Can you work these out from the model? Positions are in its coordinate system, mm. A direction names the side the tool comes from. Coordinates: 2 decimals unless noted, no trailing zeros. Write each loop counter-clockwise with the first axis right and the second up, starting at its lowest first coordinate (ties: lowest second). Pieces come first, ordered by that corner, then holes.
```python
from build123d import *

# Parameters (mm, degrees)
CUT_EXTRUDE_START   = -20
SKETCH_2_R          = 35
CUT_EXTRUDE_1_DEPTH = 20


with BuildPart() as part:
    # Эскиз1 → Повернуть1 (revolve)
    with BuildSketch(Plane.XY, mode=Mode.PRIVATE) as revolve_1_sk:
        Polygon((0, 0), (-35, 0), (-35, 15), (-120, 15), (-120, 10), (-40, 10), (-40, -30), (0, -30), align=None)
    revolve(revolve_1_sk.sketch.rotate(Axis((0, -30, 0), (0, 1, 0)), 270), axis=Axis((0, -30, 0), (0, 1, 0)))

    # Эскиз2 → Вырез-Вытянуть1 (cut)
    with BuildSketch(Plane.XZ.offset(30).offset(CUT_EXTRUDE_START)):
        with Locations(Location((0, 0, 0), (0, 0, 270))):
            Circle(SKETCH_2_R)
    extrude(amount=CUT_EXTRUDE_1_DEPTH, mode=Mode.SUBTRACT)


solid = part.part
```
1. If we section it at A-A, the plane y = -18: List the corners of the cut face in (x, z) for me, plus the area to 3 significant figures.
2. If we section it at D-D, the plane x = 65: List the corners of the cut face in (y, z) for me.
3. If we section it at C-C, the plane z = -4: List the corners of the cut face in (x, y) for me, plus the area to 3 significant figures.
4. Which directions (+Z, -Z, +X, -X, +Y, -Y) give clear straight access to the entire face, cutting with the end or side of a thin tool? Please do faces 4 (the face through (39.05, -10.28, 8.67)), 5 (the face through (21, 8, 28)), 6 (the face through (35.4, -30, 0.2)).
5. If we section it at B-B, the plane x = 0: List the corners of the cut face in (y, z) for me.
6. If I drill on L1, parallel to X at y = 10.25, z = 0; L2, parallel to X at y = 4, z = 0; L3, parallel to Y at x = -33, z = 3, over which ranges is the centre line in solid material (lowest first)?
7. We'd pull the mould along X, two halves only. Please class faces 1 (the face through (-5.276, 12.465, 119.884)), 2 (the face through (-2, 10, -52)), 3 (the face through (0, -10, 0)): released by +X, released by -X, zero draft, split by the parting line, or undercut.
8. I'm going to push flat-ended pins straight in: P1, Ø2, axis at y = 1.5, z = 27.5, coming from the +X side; P2, Ø8, axis at x = 38.5, y = -6, coming from the +Z side; P3, Ø6, axis at x = 6.5, y = 6.5, coming from the +Z side. Where does each tip first touch, or does it pass through?
Answers:
1. outline: circle Ø80 at (0, 0); hole circle Ø70 at (0, 0)
1. area: 1,180 mm2
2. outline: (10, -100.87) - (15, -100.87) - (15, 100.87) - (10, 100.87) - close
3. outline: (-119.93, 10) - (-39.8, 10) - (-39.8, -30) - (-34.77, -30) - (-34.77, -10) - (34.77, -10) - (34.77, -30) - (39.8, -30) - (39.8, 10) - (119.93, 10) - (119.93, 15) - (34.77, 15) - (34.77, 0) - (-34.77, 0) - (-34.77, 15) - (-119.93, 15) - close
3. area: 1,950 mm2
4. face 4: -Y
4. face 5: +Y
4. face 6: +Z, -Z, +X, -X, -Y
5. outline: (-30, -40) - (10, -40) - (10, -120) - (15, -120) - (15, -35) - (0, -35) - (0, 35) - (15, 35) - (15, 120) - (10, 120) - (10, 40) - (-30, 40) - (-30, 35) - (-10, 35) - (-10, -35) - (-30, -35) - close
6. L1: x = -120 to -35, 35 to 120
6. L2: x = -40 to -35, 35 to 40
6. L3: y = -10 to 0
7. face 1: split by the parting line
7. face 2: zero draft
7. face 3: undercut
8. P1: stops at x = 29.96
8. P2: stops at z = 20.24
8. P3: stops at z = 39.85
